Here's how the part is built. I have some questions about the finished solid (model axes, mm). A direction names the side the tool comes from. Round coordinates to 2 decimals unless told otherwise and drop trailing zeros. Write each loop counter-clockwise with the first axis right and the second up, starting at its lowest first coordinate (ties: lowest second). Pieces come first, ordered by that corner, then holes. Notation, with made-up numbers: (50.25, 73.25) -> (99.25, 73.25) arc R34 ccw to (99.25, 108.25) -> close; hole circle Ø2 at (86.5, 40). An arc over 180 degrees is marked (long way). Put each result on its own line as item: value. Start each with the question number.
1. Suppose I cut it at A-A (x = 72.5). Please give me the cut outline in (y, z), then the cut area to 3 significant figures.
2. For pin 1 (0.9 mm diameter, centred on x = -8.5, y = 1.5, fed in from -Z); pin 2 (0.9 mm diameter, centred on x = -56.5, y = 2, fed in from -Z) (3 decimals); pin 3 (5 mm diameter, centred on x = -72.5, z = -21.5, fed in from +Y), each with a flat end and sliding along its axis, tell me the tip position at first contact or that it passes through.
3. Suppose I cut it at B-B (z = 2). Count the separate pieces of the cut face and the enclosed holes in it, then the cut area to 3 significant figures.
4. Which directions (+Z, -Z, +X, -X, +Y, -Y) give clear straight access to the entire face, cutting with the end or side of a thin tool? Please do faces 3 (the face through (-72, 1, 26)), 4 (the face through (-54.5, 2, 0)), 5 (the face through (1, 1, 16)).
5. We'd pull the mould along X, two halves only. Please class faces 1 (the face through (-50, 2, 8)), 2 (the face through (72, 1, -26)): +X half, -X half, draft (parallel to the pull), parting line (faces both ways), or undercut.
6. I need wall thicknesses on probe 1 along Z at (x, y) = (-72.5, 1.85); probe 2 along X at (y, z) = (0.6, -15); probe 3 along Z at (x, y) = (-58.5, 2.8). Which ranges of each line are inside material? Lowest first, please. Write a range as from..to.
7. Suppose I cut it at D-D (x = 17). Please give me the cut outline in (y, z).
```python
from build123d import *

# Parameters (mm, degrees)
EXTRUDE_2_DEPTH       = 3
HOLE_WIZARD_3_0_3_6_D = 3
SKETCH_9_W            = 10
SKETCH_9_H            = 22
SKETCH_9_H_2          = 16
CUT_EXTRUDE_1_DEPTH   = 3
FILLET_1_R            = 2


with BuildPart() as part:
    # Sketch 1 → Extrude 2 (new body)
    with BuildSketch(Plane(origin=(0, 0, 0), x_dir=(1, 0, 0), z_dir=(0, 1, 0))):
        Polygon((-82.5, 26), (-62.5, 26), (-42.5, 16), (42.5, 16), (62.5, 26), (82.5, 26), (82.5, -26), (62.5, -26), (42.5, -16), (-42.5, -16), (-62.5, -26), (-82.5, -26), align=None)
    extrude(amount=EXTRUDE_2_DEPTH)

    # Hole Wizard 3.0 _3_ _6 (through all)
    with Locations(Plane(origin=(-72.5, 3, -21.5), x_dir=(0, 0, 1), z_dir=(0, 1, 0))):
        with Locations((0, 0), (0, 145), (43, 145), (43, 0)):
            Hole(HOLE_WIZARD_3_0_3_6_D / 2)

    # Sketch 9 → Cut-Extrude 1 (cut)
    with BuildSketch(Plane(origin=(0, 3, 0), x_dir=(1, 0, 0), z_dir=(0, 1, 0))):
        with Locations((-72.5, 0)):
            Rectangle(SKETCH_9_W, SKETCH_9_H)
        with Locations((72.5, 0)):
            Rectangle(SKETCH_9_W, SKETCH_9_H)
        Polygon((-62.5, 21.455387521), (-62.5, 12.455387521), (-44.5, 12.455387521), align=None)
        Polygon((44.5, 12.5), (62.5, 21.5), (62.5, 12.5), align=None)
        Polygon((62.5, -12.5), (44.5, -12.5), (62.5, -21.5), align=None)
        Polygon((-44.5, -12.5), (-62.5, -21.5), (-62.5, -12.5), align=None)
        with Locations((-49.5, 0)):
            Rectangle(SKETCH_9_W, SKETCH_9_H_2)
        with Locations((-29.7, 0)):
            Rectangle(SKETCH_9_W, SKETCH_9_H_2)
        with Locations((-9.9, 0)):
            Rectangle(SKETCH_9_W, SKETCH_9_H_2)
        with Locations((29.7, 0)):
            Rectangle(SKETCH_9_W, SKETCH_9_H_2)
        with Locations((49.5, 0)):
            Rectangle(SKETCH_9_W, SKETCH_9_H_2)
        with Locations((9.9, 0)):
            Rectangle(SKETCH_9_W, SKETCH_9_H_2)
    extrude(amount=-CUT_EXTRUDE_1_DEPTH, mode=Mode.SUBTRACT)

    # Fillet 1
    fillet_1_edges = [part.edges().sort_by_distance(p)[0] for p in [
        (-67.5, 1.5, -11),
        (-67.5, 1.5, 11),
        (-77.5, 1.5, 11),
        (-77.5, 1.5, -11),
        (14.9, 1.5, 8),
        (4.9, 1.5, 8),
        (4.9, 1.5, -8),
        (14.9, 1.5, -8),
        (34.7, 1.5, 8),
        (24.7, 1.5, 8),
        (24.7, 1.5, -8),
        (34.7, 1.5, -8),
        (54.5, 1.5, -8),
        (54.5, 1.5, 8),
        (44.5, 1.5, 8),
        (44.5, 1.5, -8),
        (62.5, 1.5, -12.5),
        (44.5, 1.5, -12.5),
        (62.5, 1.5, -21.5),
        (62.5, 1.5, 12.5),
        (62.5, 1.5, 21.5),
        (44.5, 1.5, 12.5),
        (-62.5, 1.5, -21.455387521),
        (-44.5, 1.5, -12.455387521),
        (-62.5, 1.5, -12.455387521),
        (77.5, 1.5, -11),
        (77.5, 1.5, 11),
        (67.5, 1.5, 11),
        (67.5, 1.5, -11),
        (-62.5, 1.5, 12.5),
        (-44.5, 1.5, 12.5),
        (-62.5, 1.5, 21.5),
        (-44.5, 1.5, -8),
        (-44.5, 1.5, 8),
        (-54.5, 1.5, 8),
        (-54.5, 1.5, -8),
        (-24.7, 1.5, 8),
        (-34.7, 1.5, 8),
        (-34.7, 1.5, -8),
        (-24.7, 1.5, -8),
        (-4.9, 1.5, 8),
        (-14.9, 1.5, 8),
        (-14.9, 1.5, -8),
        (-4.9, 1.5, -8),
    ]]
    fillet(fillet_1_edges, radius=FILLET_1_R)


solid = part.part
```
Verdict:
1. outline: (0, -26) -> (3, -26) -> (3, -23) -> (0, -23) -> close; (0, -20) -> (3, -20) -> (3, -11) -> (0, -11) -> close; (0, 11) -> (3, 11) -> (3, 20) -> (0, 20) -> close; (0, 23) -> (3, 23) -> (3, 26) -> (0, 26) -> close
1. area: 72.0 mm^2
2. pin 1: stops at z = -16
2. pin 2: stops at z = -23.225
2. pin 3: stops at y = 3
3. separate pieces: 9
3. enclosed holes: 0
3. area: 255 mm^2
4. face 3: +Z, +X, -X, +Y, -Y
4. face 4: +Y, -Y
4. face 5: +Z, +Y, -Y
5. face 1: undercut
5. face 2: draft
6. probe 1: z = -26..-23, -20..-11, 11..20, 23..26
6. probe 2: x = -82.5..-62.5, -51.05..51.04, 62.5..82.5
6. probe 3: z = -24..-19.46, -12.46..12.5, 19.5..24
7. outline: (0, -16) -> (3, -16) -> (3, 16) -> (0, 16) -> close
